Geometry check sheet. Reference: the model listing, model coordinates, mm. Give positions to 0.01 mm unless a question says otherwise; leave off trailing zeros. Order: outer loops, then holes, each group sorted by start corner. A loop starts at its lowest first (then second) coordinate and runs counter-clockwise, first axis right, second up.
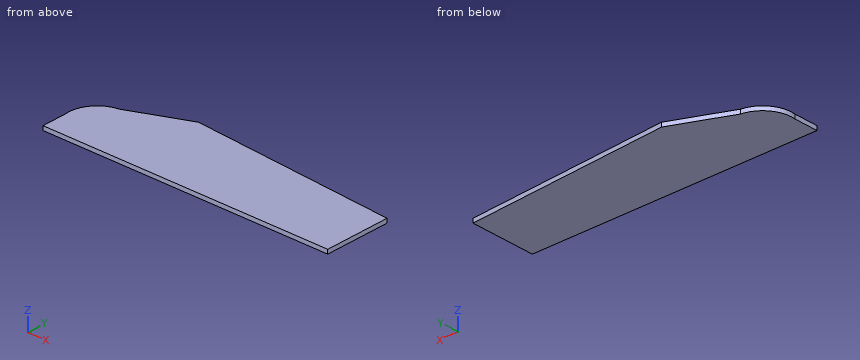
from build123d import *

# Parameters (mm, degrees)
BOSS_EXTRU_1_DEPTH = 5


with BuildPart() as part:
    # Esquisse1 → Boss.-Extru.1 (new body)
    with BuildSketch(Plane.XY):
        with BuildLine():
            Line((0, 0), (350, 0))
            Line((350, 0), (350, 80))
            Line((350, 80), (100, 100))
            Line((100, 100), (30, 70))
            ThreePointArc((30, 70), (6.595917942, 56.303061543), (0, 30))
            Line((0, 30), (0, 0))
        make_face()
    extrude(amount=BOSS_EXTRU_1_DEPTH)


solid = part.part
Item 1: Sectioned sample at B-B (x = 197.5). Enter the section's corners in (y, z).
Reported:
outline: (0, 0) - (92.2, 0) - (92.2, 5) - (0, 5) - close
Item 2: Gauge pin test, flat end, axial feed: pin 1 (1 mm diameter, centred on y = 87.5, z = 2, fed in from -X). Record the tip position at first contact, or that the pin passes through.
Reported:
pin 1: stops at x = 69.67
Item 3: Sectioned sample at A-A (z = 2.45). Enter the section's corners in (x, y), and give its area (3 significant figures).
Reported:
outline: (0, 0) - (350, 0) - (350, 80) - (100, 100) - (30, 70) arc R35 ccw to (0, 30) - close
area: 30,300 mm2
Item 4: Sectioned sample at C-C (y = 93). Enter the section's corners in (x, z).
Reported:
outline: (83.67, 0) - (187.5, 0) - (187.5, 5) - (83.67, 5) - close
Item 5: Scan lines: L1, parallel to X at y = 9.5, z = 2.6; L2, parallel to X at y = 34, z = 2.9; L3, parallel to Y at x = 55.5, z = 2.3. Record each from-to range of solid material in increasing order.
Reported:
L1: x = 0 to 350
L2: x = -0.38 to 350
L3: y = 0 to 80.93
